```python
from build123d import *

# Parameters (mm, degrees)
F0_R     = 2.5
F1_DEPTH = 5
F2_R     = 2.5
F3_DEPTH = 25


with BuildPart() as f1:
    # F0 (on Top) → F1 (new body)
    with BuildSketch(Plane.XY):
        with BuildLine():
            ThreePointArc((193, -7.5), (200.5, 0), (193, 7.5))
            Line((193, 7.5), (-193, 7.5))
            ThreePointArc((-193, 7.5), (-200.5, 0), (-193, -7.5))
            Line((-193, -7.5), (193, -7.5))
        make_face()
        with Locations((-193, 0)):
            Circle(F0_R, mode=Mode.SUBTRACT)
        Circle(F0_R, mode=Mode.SUBTRACT)
        with Locations((193, 0)):
            Circle(F0_R, mode=Mode.SUBTRACT)
    extrude(amount=F1_DEPTH)

    # F2 (on face) → F3 (cut)
    with BuildSketch(Plane.XY.offset(5)):
        Circle(F2_R)
        with BuildLine():
            ThreePointArc((0, 7.5), (5.303301, 5.303301), (7.5, 0))
            ThreePointArc((7.5, 0), (5.303301, -5.303301), (0, -7.5))
            Line((0, -7.5), (193, -7.5))
            ThreePointArc((193, -7.5), (200.5, 0), (193, 7.5))
            Line((193, 7.5), (0, 7.5))
        make_face()
        with Locations((193, 0)):
            Circle(F2_R, mode=Mode.SUBTRACT)
    extrude(amount=-F3_DEPTH, mode=Mode.SUBTRACT)


solid = f1.part
```
CAD build for the part. Positions are in the model's coordinates, mm. Round coordinates to 2 decimals unless told otherwise and drop trailing zeros. Loops run counter-clockwise (first coordinate to the right, second up) from the corner with the lowest first, then second, coordinate; pieces in that order, holes last. Notation, with made-up numbers: M 5.5,16.25 L 57.5,16.25 A14 ccw 57.5,34.25 Z; hole C -37,49 d8. An arc over 180 degrees is marked long. Use a Markdown table: item, result. Add a question column.
(1) Drill centre lines: line 1 (X direction, y = 0.25, z = 2.45); line 2 (Y direction, x = -193, z = 2.2); line 3 (X direction, y = 2.25, z = 0.4). Where is each one in solid material? Low to high.
(2) Pull direction X, two halves, no side cores. Call faces 1 (the face through (-200.5, 0.16, 2.46)), 2 (the face through (-0.54, -2.44, 2.46)), 3 (the face through (-98, 0, 0)): +X half, -X half, draft (parallel to the pull), parting line (faces both ways), or undercut.
(3) Flat gauge pins, fed straight in: pin 1 (1 mm diameter, centred on y = -5.5, z = 1, fed in from +X); pin 2 (3 mm diameter, centred on y = 4, z = 4.5, fed in from +X); pin 3 (1 mm diameter, centred on y = 1.5, z = 3, fed in from +X). Where does each tip first touch, or does it go through?
(4) Cut at C-C (y = 5.25). Give the cut face in (x, z).
(5) Cut at B-B (y = -5.5). Give the cut face in (x, z), and give its area (3 significant figures).
(6) Cut at A-A (z = 2.2). Give the cut face in (x, y).
Geometry says:
| question | item | result |
|---|---|---|
| 1 | line 1 | x = -200.5 to -195.49, -190.51 to -2.49, 2.49 to 7.5 |
| 1 | line 2 | y = -7.5 to -2.5, 2.5 to 7.5 |
| 1 | line 3 | x = -200.15 to -194.09, -191.91 to -1.09, 1.09 to 7.15 |
| 2 | face 1 | -X half |
| 2 | face 2 | undercut |
| 2 | face 3 | draft |
| 3 | pin 1 | stops at x = 5.59 |
| 3 | pin 2 | stops at x = 7.07 |
| 3 | pin 3 | stops at x = 7.43 |
| 4 | outline | M -198.36,0 L 5.36,0 L 5.36,5 L -198.36,5 Z |
| 5 | outline | M -198.1,0 L 5.1,0 L 5.1,5 L -198.1,5 Z |
| 5 | area | 1,020 mm² |
| 6 | outline | M -193,-7.5 L 0,-7.5 A7.5 ccw 0,7.5 L -193,7.5 A7.5 ccw Z; hole C -193,0 d5; hole C 0,0 d5 |
